The listing builds one solid part. Answer for the finished solid, in the listing's coordinates (mm). A direction names the side the tool comes from. Round coordinates to 2 decimals unless told otherwise and drop trailing zeros. Order: outer loops, then holes, each group sorted by start corner. A loop starts at its lowest first (then second) coordinate and runs counter-clockwise, first axis right, second up. Notation, with made-up numbers: (20.5, 43.5) - (52.5, 43.5) arc R16 cw to (52.5, 56.5) - close; hole circle Ø2 at (13.25, 14). An arc over 180 degrees is marked (long way). One line per item, written item: value. Start each with the question number.
1. Straight lines are drawn through the part: line 1 (X direction, y = 29.75, z = 9.95); line 2 (X direction, y = 2, z = 9.5); line 3 (X direction, y = -10.5, z = 7.5). For each, find the intervals that lie inside material, in ascending order.
2. For a pull along X with two mould halves and no side action, classify faces 1 (the flat face through (21, 17, 2)), 2 (the cylindrical face through (-21.76, 32.8, 5.92)), 3 (the cylindrical face through (-8.4, -13.8, 4.8)) as released by +X, released by -X, zero draft, split by the parting line, or undercut.
3. Section B-B, the plane x = 2 is taken. Give the vertices of the cut face in (y, z), then the cut area to 3 significant figures.
4. Flat-ended cylindrical pins translate along their axes: P1, Ø8, axis at x = 13.5, y = -8.75, coming from the -Z side; P2, Ø3.5, axis at x = 19.75, y = 15.5, coming from the -Z side; P3, Ø1.8, axis at y = 31, z = 4.5, coming from the -X side. Find the tip coordinate at first contact, or state that the pin passes through.
5. Section A-A, the plane y = 9.5 is taken. Give the vertices of the cut face in (x, z).
6. A tool of negligible diameter and unlimited length cuts with its end or side. For faces 4 (the cylindrical face through (-16.497, -8.618, 4.511)), 5 (the flat face through (0, 27, 0)), 6 (the flat face through (0, 28.5, 7)), 7 (the flat face through (-6.5, 30.2, 3.4)), 8 (the cylindrical face through (-15.43, 25.4, 5.92)), from which of +Z, -Z, +X, -X, +Y, -Y can it reach the whole face along a straight path? Write none if from no direction.
from build123d import *

# Parameters (mm, degrees)
BOSS_EXTRUDE1_DEPTH        = 12
CUT_EXTRUDE1_REACH         = 44.644
SKETCH3_R                  = 1.6
SKETCH6_W                  = 10
SKETCH6_H                  = 5
CUT_EXTRUDE3_DEPTH         = 9
CUT_EXTRUDE4_DEPTH         = 12.5
CUT_EXTRUDE5_START         = -23.5
CUT_EXTRUDE5_OUTLINE_R     = 3
CUT_EXTRUDE5_DEPTH         = 15.5
BOSS_EXTRUDE4_START        = -23.5
BOSS_EXTRUDE4_DEPTH        = 47
PIVOTSCREWHEADCUTOUT_START = -23.5
SKETCH10_R                 = 3
PIVOTSCREWHEADCUTOUT_DEPTH = 13
CUT_EXTRUDE2_START         = 8.5
SKETCH4_R                  = 3
CUT_EXTRUDE2_DEPTH         = 52.143874282
CUT_EXTRUDE10_START        = 10
SKETCH16_R                 = 3
CUT_EXTRUDE10_DEPTH        = 160.510325132
CUT_EXTRUDE7_START         = -23.5
CUT_EXTRUDE7_DEPTH         = 37
FILLET1_R                  = 3.5
CUT_EXTRUDE9_DEPTH         = 6.25


# Read off the part's stored shape, not the designer's step: Cut-Extrude5
with BuildPart() as part:
    # Sketch2 → Boss-Extrude1 (new body)
    with BuildSketch(Plane.XY):
        with BuildLine():
            Line((23.5, -8.75), (23.5, 29.5))
            ThreePointArc((23.5, 29.5), (22.328427125, 32.328427125), (19.5, 33.5))
            Line((19.5, 33.5), (-19.5, 33.5))
            ThreePointArc((-19.5, 33.5), (-22.328427125, 32.328427125), (-23.5, 29.5))
            Line((-23.5, 29.5), (-23.5, -8.75))
            Line((-23.5, -8.75), (-23.5, -12.5))
            Line((-23.5, -12.5), (-19.499997491, -12.5))
            Line((-19.499997491, -12.5), (19.531687848, -12.5))
            Line((19.531687848, -12.5), (23.5, -12.5))
            Line((23.5, -12.5), (23.5, -8.75))
        make_face()
        with BuildLine():
            Line((-16, -3), (-16, 24))
            ThreePointArc((-16, 24), (-15.414213562, 25.414213562), (-14, 26))
            Line((-14, 26), (14, 26))
            ThreePointArc((14, 26), (15.414213562, 25.414213562), (16, 24))
            Line((16, 24), (16, -3))
            ThreePointArc((16, -3), (15.414213562, -4.414213562), (14, -5))
            Line((14, -5), (-14, -5))
            ThreePointArc((-14, -5), (-15.414213562, -4.414213562), (-16, -3))
        make_face(mode=Mode.SUBTRACT)
    extrude(amount=BOSS_EXTRUDE1_DEPTH)

    # Sketch3 → Cut-Extrude1 (cut, up to next)
    with BuildSketch(Plane.XY, mode=Mode.PRIVATE) as cut_extrude1_sk1:
        with Locations((-13.5, 29.75)):
            Circle(SKETCH3_R)
    cut_extrude1_tool1 = extrude(cut_extrude1_sk1.sketch, amount=CUT_EXTRUDE1_REACH, mode=Mode.PRIVATE) & part.part
    # Sketch3 → Cut-Extrude1 (cut, up to next)
    with BuildSketch(Plane.XY, mode=Mode.PRIVATE) as cut_extrude1_sk2:
        with Locations((13.5, 29.75)):
            Circle(SKETCH3_R)
    cut_extrude1_tool2 = extrude(cut_extrude1_sk2.sketch, amount=CUT_EXTRUDE1_REACH, mode=Mode.PRIVATE) & part.part
    # Sketch3 → Cut-Extrude1 (cut, up to next)
    with BuildSketch(Plane.XY, mode=Mode.PRIVATE) as cut_extrude1_sk3:
        with Locations((19.75, 15.5)):
            Circle(SKETCH3_R)
    cut_extrude1_tool3 = extrude(cut_extrude1_sk3.sketch, amount=CUT_EXTRUDE1_REACH, mode=Mode.PRIVATE) & part.part
    # Sketch3 → Cut-Extrude1 (cut, up to next)
    with BuildSketch(Plane.XY, mode=Mode.PRIVATE) as cut_extrude1_sk4:
        with Locations((-19.75, 15.5)):
            Circle(SKETCH3_R)
    cut_extrude1_tool4 = extrude(cut_extrude1_sk4.sketch, amount=CUT_EXTRUDE1_REACH, mode=Mode.PRIVATE) & part.part
    # Sketch3 → Cut-Extrude1 (cut, up to next)
    with BuildSketch(Plane.XY, mode=Mode.PRIVATE) as cut_extrude1_sk5:
        with Locations((-13.5, -8.75)):
            Circle(SKETCH3_R)
    cut_extrude1_tool5 = extrude(cut_extrude1_sk5.sketch, amount=CUT_EXTRUDE1_REACH, mode=Mode.PRIVATE) & part.part
    # Sketch3 → Cut-Extrude1 (cut, up to next)
    with BuildSketch(Plane.XY, mode=Mode.PRIVATE) as cut_extrude1_sk6:
        with Locations((13.5, -8.75)):
            Circle(SKETCH3_R)
    cut_extrude1_tool6 = extrude(cut_extrude1_sk6.sketch, amount=CUT_EXTRUDE1_REACH, mode=Mode.PRIVATE) & part.part
    add(cut_extrude1_tool1.solids().sort_by_distance((-13.5, 29.75, 0))[0], mode=Mode.SUBTRACT)
    add(cut_extrude1_tool2.solids().sort_by_distance((13.5, 29.75, 0))[0], mode=Mode.SUBTRACT)
    add(cut_extrude1_tool3.solids().sort_by_distance((19.75, 15.5, 0))[0], mode=Mode.SUBTRACT)
    add(cut_extrude1_tool4.solids().sort_by_distance((-19.75, 15.5, 0))[0], mode=Mode.SUBTRACT)
    add(cut_extrude1_tool5.solids().sort_by_distance((-13.5, -8.75, 0))[0], mode=Mode.SUBTRACT)
    add(cut_extrude1_tool6.solids().sort_by_distance((13.5, -8.75, 0))[0], mode=Mode.SUBTRACT)

    # Sketch6 → Cut-Extrude3 (cut)
    with BuildSketch(Plane.XY):
        with Locations((0, 31)):
            Rectangle(SKETCH6_W, SKETCH6_H)
    extrude(amount=CUT_EXTRUDE3_DEPTH, mode=Mode.SUBTRACT)

    # Sketch7 → Cut-Extrude4 (cut, symmetric)
    with BuildSketch(Plane(origin=(0, 0, 0), x_dir=(0, 0, -1), z_dir=(1, 0, 0))):
        with BuildLine():
            Line((-4, 30.8), (-2.7, 29.5))
            Line((-2.7, 29.5), (-4, 28.2))
            ThreePointArc((-4, 28.2), (-5.3, 29.5), (-4, 30.8))
        make_face()
    extrude(amount=CUT_EXTRUDE4_DEPTH, both=True, mode=Mode.SUBTRACT)

    # Cut-Extrude5 outline → Cut-Extrude5 (cut)
    with BuildSketch(Plane(origin=(0, 0, 0), x_dir=(0, 0, -1), z_dir=(1, 0, 0)).offset(CUT_EXTRUDE5_START)):
        with Locations((-4, 29.5)):
            Circle(CUT_EXTRUDE5_OUTLINE_R)
    extrude(amount=CUT_EXTRUDE5_DEPTH, mode=Mode.SUBTRACT)

    # Sketch14 → Boss-Extrude4 (add)
    with BuildSketch(Plane(origin=(0, 0, 0), x_dir=(0, 0, -1), z_dir=(1, 0, 0)).offset(BOSS_EXTRUDE4_START)):
        with BuildLine():
            Line((-3.5, -19.55), (-12, -12.5))
            Line((-12, -12.5), (0, -12.5))
            Line((0, -12.5), (0, -9.125067568))
            ThreePointArc((0, -9.125067568), (1.998391042, -15.595994569), (-3.5, -19.55))
        make_face()
    extrude(amount=BOSS_EXTRUDE4_DEPTH)

    # Sketch10 → PivotScrewHeadCutout (cut)
    with BuildSketch(Plane(origin=(0, 0, 0), x_dir=(0, 0, -1), z_dir=(1, 0, 0)).offset(PIVOTSCREWHEADCUTOUT_START)):
        with Locations(Location((-3.5, -13.75, 0), (0, 0, 180))):
            Circle(SKETCH10_R)
    extrude(amount=PIVOTSCREWHEADCUTOUT_DEPTH, mode=Mode.SUBTRACT)

    # Sketch4 → Cut-Extrude2 (cut, through all)
    with BuildSketch(Plane.XY.offset(CUT_EXTRUDE2_START)):
        with Locations((-13.5, 29.75)):
            Circle(SKETCH4_R)
        with Locations((-13.5, -8.75)):
            Circle(SKETCH4_R)
    extrude(amount=-CUT_EXTRUDE2_DEPTH, mode=Mode.SUBTRACT)

    # Sketch16 → Cut-Extrude10 (cut, through all)
    with BuildSketch(Plane(origin=(67.926630299, -108.522644494, 12), x_dir=(-1, 0, 0), z_dir=(0, 0, -1)).offset(CUT_EXTRUDE10_START)):
        with Locations(Location((54.426630299, 138.272644494, 0), (0, 0, 180))):
            Circle(SKETCH16_R)
        with Locations(Location((87.676630299, 124.022644494, 0), (0, 0, 180))):
            Circle(SKETCH16_R)
        with Locations(Location((54.426630299, 99.772644494, 0), (0, 0, 187.18205644))):
            Circle(SKETCH16_R)
        with Locations(Location((48.176630299, 124.022644494, 0), (0, 0, 180))):
            Circle(SKETCH16_R)
    extrude(amount=CUT_EXTRUDE10_DEPTH, mode=Mode.SUBTRACT)

    # Sketch9 → Cut-Extrude7 (cut)
    with BuildSketch(Plane(origin=(0, 0, 0), x_dir=(0, 0, -1), z_dir=(1, 0, 0)).offset(CUT_EXTRUDE7_START)):
        with BuildLine():
            Line((-3.5, -12.45), (-2.2, -13.75))
            Line((-2.2, -13.75), (-3.5, -15.05))
            ThreePointArc((-3.5, -15.05), (-4.8, -13.75), (-3.5, -12.45))
        make_face()
    extrude(amount=CUT_EXTRUDE7_DEPTH, mode=Mode.SUBTRACT)

    # Fillet1
    # the kernel refuses this fillet: 3.5 mm, written as the material it takes off along each edge
    with BuildSketch(Plane(origin=(23.5, -25.136011381, -3.234907338), x_dir=(0, 0.769703695807885, -0.6384013006406574), z_dir=(0, 0.6384013006406574, 0.769703695807885)), Plane(origin=(-23.5, -25.136011381, -3.234907338), x_dir=(1, 0, 0), z_dir=(0, 0.6384013006406574, 0.769703695807885))) as fillet1_piece_1:
        with BuildLine():
            CenterArc((FILLET1_R, FILLET1_R), FILLET1_R, 180, 90)
            Line((0, FILLET1_R), (0, 0))
            Line((0, 0), (FILLET1_R, 0))
        make_face()
    extrude(amount=28.543210584, mode=Mode.SUBTRACT)

    # Sketch15 → Cut-Extrude9 (cut, symmetric)
    with BuildSketch(Plane(origin=(0, 0, 0), x_dir=(0, 0, -1), z_dir=(1, 0, 0))):
        with BuildLine():
            Line((-10.3, -13.75), (-10.3, -20.55))
            Line((-10.3, -20.55), (-3.5, -20.55))
            ThreePointArc((-3.5, -20.55), (1.308326112, -8.941673888), (-10.3, -13.75))
        make_face()
    extrude(amount=CUT_EXTRUDE9_DEPTH, both=True, mode=Mode.SUBTRACT)


solid = part.part
Answer list:
1. line 1: x = -23.49 to -15.1, -11.9 to 11.9, 15.1 to 23.49
1. line 2: x = -23.5 to -16, 16 to 23.5
1. line 3: x = -23.5 to -15.94, -11.06 to -6.25, 6.25 to 23.5
2. face 1: undercut
2. face 2: released by -X
2. face 3: zero draft
3. outline: (-13.91, 10.3) - (-13.75, 10.3) arc R6.8 cw to (-7.92, 0) - (-5, 0) - (-5, 12) - (-12.5, 12) - close; (26, 0) - (28.5, 0) - (28.5, 3.7) - (28.2, 4) arc R1.3 cw to (28.5, 4.83) - (28.5, 9) - (33.5, 9) - (33.5, 12) - (26, 12) - close
3. area: 89.8 mm²
4. P1: stops at z = -2.21
4. P2: stops at z = 2
4. P3: stops at x = -8
5. outline: (-23.5, 0) - (-16, 0) - (-16, 12) - (-23.5, 12) - close; (16, 0) - (23.5, 0) - (23.5, 12) - (16, 12) - close
6. face 4: -Z
6. face 5: -Z, +X, -X, +Y
6. face 6: -Z, +Y
6. face 7: -X
6. face 8: +Z, -Z
